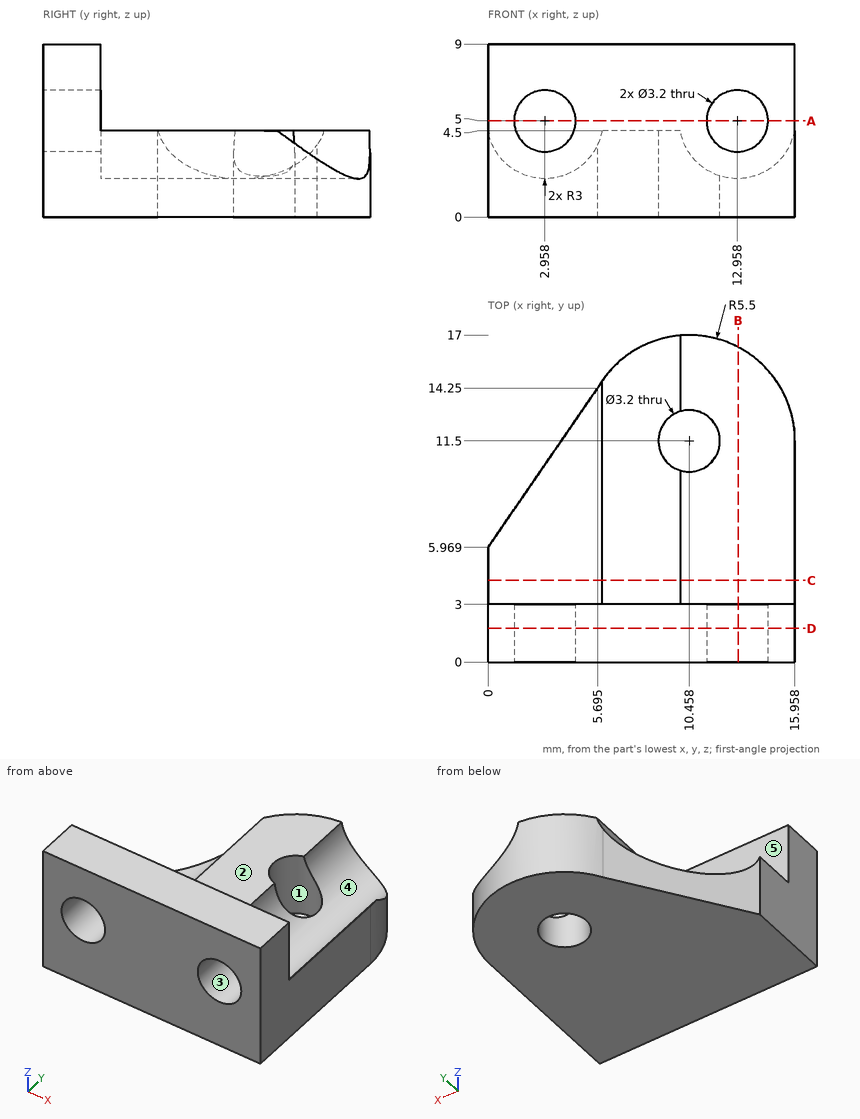
Part print with two shaded views. Sizes in mm from the minimum x, y, z corner. A direction names the side the tool comes from. Round coordinates to 2 decimals unless told otherwise and drop trailing zeros. Loops run counter-clockwise (first coordinate to the right, second up) from the corner with the lowest first, then second, coordinate; pieces in that order, holes last.
1. Two-plate mould, pull along Z, no slides. Class the marked faces 3, 4 and 5: pulls with the +Z half, pulls with the -Z half, needs draft (parallel to the pull), parting line crosses it, or undercut.
Solutions:
face 3: undercut
face 4: pulls with the +Z half
face 5: needs draft
2. Slice it at A-A (z = 5). Give the cut face in (x, y), and give its area (3 significant figures).
Solutions:
outline: (0, 0) - (1.36, 0) - (1.36, 3) - (0, 3) - close; (4.56, 0) - (11.36, 0) - (11.36, 3) - (4.56, 3) - close; (14.56, 0) - (15.96, 0) - (15.96, 3) - (14.56, 3) - close
area: 28.7 mm2
3. Slice it at C-C (y = 4.25). Give the cut face in (x, z), and give its area (3 significant figures).
Solutions:
outline: (0, 0) - (15.96, 0) - (15.96, 4.5) - (15.92, 4.5) arc R3 cw to (10, 4.5) - (5.92, 4.5) arc R3 cw to (0, 4.5) - close
area: 49.5 mm2
4. Slice it at D-D (y = 1.75). Give the cut face in (x, z).
Solutions:
outline: (0, 0) - (15.96, 0) - (15.96, 9) - (0, 9) - close; hole circle Ø3.2 at (2.96, 5); hole circle Ø3.2 at (12.96, 5)
5. 3-axis set-ups, long thin cutter, end or side, ignore diameter. For the marked faces 1 and 2: which of +Z, -Z, +X, -X, +Y, -Y reach the whole face in a straight line?
Solutions:
face 1: +Z, -Z
face 2: +Z, +X, -X, +Y
6. Slice it at B-B (x = 13). Give the cut face in (y, z).
Solutions:
outline: (0, 0) - (16.38, 0) - (16.38, 2) - (3, 2) - (3, 3.4) - (0, 3.4) - close; (0, 6.6) - (3, 6.6) - (3, 9) - (0, 9) - close
7. Drill centre lines: line 1 along Z through (x, y) = (6.25, 7.75); line 2 along Y through (x, z) = (14.75, 5); line 3 along X through (y, z) = (11, 3.25) (1 decimal). Where is each one in solid material? Low to high.
Solutions:
line 1: z = 0 to 4.5
line 2: y = 0 to 3
line 3: x = 5.4 to 8.9, 15.4 to 16
8. Flat gauge pins, fed straight in: pin 1 (5 mm diameter, centred on x = 7.5, z = 7.5, fed in from +Y); pin 2 (8 mm diameter, centred on x = 8.5, y = 15, fed in from +Z); pin 3 (1 mm diameter, centred on x = 11, y = 5, fed in from +Z). Where does each tip first touch, or does it go through?
Solutions:
pin 1: stops at y = 3
pin 2: stops at z = 4.5
pin 3: stops at z = 3.28
